from build123d import *

# Parameters (mm, degrees)
PAD_DEPTH       = 8
SKETCH001_W     = 10
SKETCH001_H     = 10
POCKET_DEPTH    = 9.1
POCKET006_DEPTH = 4.5
SKETCH016_W     = 1.5
SKETCH016_H     = 1.5
SKETCH016_H_2   = 2.241798
POCKET007_DEPTH = 8.001


with BuildPart() as part:
    # Sketch → Pad (new body)
    with BuildSketch(Plane.XY):
        Polygon((1.5, 9), (15, 9), (15, 4.5), (19, 4.5), (19, -4.5), (15, -4.5), (15, -9), (1.5, -9), (1.5, -10.5), (-3, -10.5), (-3, 10.5), (1.5, 10.5), align=None)
    extrude(amount=PAD_DEPTH)

    # Sketch001 → Pocket (cut, symmetric)
    with BuildSketch(Plane.XZ):
        with Locations((-5, 10)):
            Rectangle(SKETCH001_W, SKETCH001_H)
    extrude(amount=POCKET_DEPTH, both=True, mode=Mode.SUBTRACT)

    # Sketch015 → Pocket006 (cut)
    with BuildSketch(Plane.XY):
        Polygon((12, 10), (13.5, 10), (13.5, 3), (16.5, 3), (16.5, 10), (18, 10), (18, -10), (16.5, -10), (16.5, -3), (13.5, -3), (13.5, -10), (12, -10), align=None)
    extrude(amount=POCKET006_DEPTH, mode=Mode.SUBTRACT)

    # Sketch016 → Pocket007 (cut, through all)
    with BuildSketch(Plane.XY):
        with Locations((17.251662, 4.766245)):
            Rectangle(SKETCH016_W, SKETCH016_H)
        with Locations((17.251662, -5.137144)):
            Rectangle(SKETCH016_W, SKETCH016_H_2)
    extrude(amount=POCKET007_DEPTH, mode=Mode.SUBTRACT)


solid = part.part
CAD build for the part. Positions are in the model's coordinates, mm. A direction names the side the tool comes from. Coordinates: 2 decimals unless noted, no trailing zeros. Loops run counter-clockwise (first coordinate to the right, second up) from the corner with the lowest first, then second, coordinate; pieces in that order, holes last. Notation, with made-up numbers: (-20.5, 10) -> (11.5, 10) arc R20 cw to (11.5, 29) -> close; hole circle Ø5 at (11, 63). An arc over 180 degrees is marked (long way). One line per item, written item: value.
1. Drill centre lines: line 1 (X direction, y = 4.25, z = 2.25); line 2 (X direction, y = 6.75, z = 3.25); line 3 (X direction, y = 1.75, z = 1.5). Where is each one in solid material? Low to high. Write a range as [from, to].
Answers:
line 1: x = [-3, 12], [13.5, 16.5], [18, 19]
line 2: x = [-3, 12], [13.5, 15]
line 3: x = [-3, 12], [18, 19]
2. Flat gauge pins, fed straight in: P1, Ø1.7, axis at x = 15.5, z = 5.5, coming from the -Y side; P2, Ø2.5, axis at x = 15, z = 3.5, coming from the +Y side; P3, Ø1.2, axis at x = 17, z = 5, coming from the +Y side. Where does each tip first touch, or does it go through?
Answers:
P1: stops at y = -9
P2: stops at y = 9
P3: stops at y = 4.5
3. Slice it at B-B on y = 2.25. Write the cut outline in (x, z), and give its area (3 significant figures).
Answers:
outline: (-3, 0) -> (12, 0) -> (12, 4.5) -> (18, 4.5) -> (18, 0) -> (19, 0) -> (19, 8) -> (0, 8) -> (0, 5) -> (-3, 5) -> close
area: 140 mm^2
4. Pull direction Y, two halves, no side cores. Call faces 1 (the face through (1.5, -10, 4)), 2 (the face through (8, -9, 4)), 3 (the face through (0, 0, 6)): pulls with the +Y half, pulls with the -Y half, needs draft (parallel to the pull), parting line crosses it, or undercut.
Answers:
face 1: needs draft
face 2: pulls with the -Y half
face 3: undercut
5. Which spindle directions (+Z, -Z, +X, -X, +Y, -Y) get a long thin tool onto all of the face, cutting with end or side? Do faces 4 (the face through (15, 3, 2)), 5 (the face through (8, 9, 4)), 6 (the face through (12, 0, 2)). Say none if no direction does.
Answers:
face 4: -Z
face 5: +Z, -Z, +X, +Y
face 6: -Z, +Y, -Y
6. Slice it at D-D on x = -0.5. Write the cut outline in (y, z).
Answers:
outline: (-10.5, 0) -> (10.5, 0) -> (10.5, 8) -> (9.1, 8) -> (9.1, 5) -> (-9.1, 5) -> (-9.1, 8) -> (-10.5, 8) -> close
7. Slice it at A-A on z = 2.25. Give the number of separate pieces and of enclosed holes in the cut face, and give its area (3 significant figures).
Answers:
separate pieces: 4
enclosed holes: 0
area: 315 mm^2
8. Slice it at C-C on z = 5.75. Write the cut outline in (x, y).
Answers:
outline: (-3, -10.5) -> (1.5, -10.5) -> (1.5, -9) -> (15, -9) -> (15, -4.5) -> (16.5, -4.5) -> (16.5, -4.02) -> (18, -4.02) -> (18, -4.5) -> (19, -4.5) -> (19, 4.5) -> (18, 4.5) -> (18, 4.02) -> (16.5, 4.02) -> (16.5, 4.5) -> (15, 4.5) -> (15, 9) -> (1.5, 9) -> (1.5, 10.5) -> (-3, 10.5) -> (-3, 9.1) -> (0, 9.1) -> (0, -9.1) -> (-3, -9.1) -> close
